```python
from build123d import *

# Parameters (mm, degrees)
SKETCH1_R           = 3.739497694
SKETCH1_R_2         = 2.032
BOSS_EXTRUDE1_DEPTH = 6.35
SKETCH2_R           = 6.5
CUT_EXTRUDE1_DEPTH  = 3.175
FILLET1_R           = 3.175
FILLET2_R           = 0.396875


with BuildPart() as part:
    # Sketch1 → Boss-Extrude1 (new, symmetric)
    with BuildSketch(Plane(origin=(0, 0, 0), x_dir=(0, 0, -1), z_dir=(1, 0, 0))):
        with BuildLine():
            Line((-5.55625, 0), (-5.55625, 28.575))
            ThreePointArc((-5.55625, 28.575), (0, 34.13125), (5.55625, 28.575))
            Line((5.55625, 28.575), (5.55625, 0))
            ThreePointArc((5.55625, 0), (0, -5.55625), (-5.55625, 0))
        make_face()
        Circle(SKETCH1_R, mode=Mode.SUBTRACT)
        with Locations((0, 28.575)):
            Circle(SKETCH1_R_2, mode=Mode.SUBTRACT)
    extrude(amount=BOSS_EXTRUDE1_DEPTH, both=True)

    # Sketch2 → Cut-Extrude1 (cut, symmetric)
    with BuildSketch(Plane(origin=(0, 0, 0), x_dir=(0, 0, -1), z_dir=(1, 0, 0))):
        with Locations((0, 28.575)):
            Circle(SKETCH2_R)
    extrude(amount=CUT_EXTRUDE1_DEPTH, both=True, mode=Mode.SUBTRACT)

    # Fillet1
    fillet1_edges = [part.edges().sort_by_distance(p)[0] for p in [
        (0, 25.20185815, 5.55625),
        (0, 25.20185815, -5.55625),
    ]]
    fillet(fillet1_edges, radius=FILLET1_R)

    # Fillet2
    fillet2_edges = [part.edges().sort_by_distance(p)[0] for p in [
        (6.35, 34.13125, 0),
        (6.35, 14.2875, 5.55625),
        (3.175, 23.886309526, -5.55625),
        (3.175, 34.13125, 0),
        (3.175, 23.886309526, 5.55625),
        (-3.175, 23.886309526, -5.55625),
        (-3.175, 34.13125, 0),
        (-3.175, 23.886309526, 5.55625),
        (6.35, -5.55625, 0),
        (-6.35, 14.2875, 5.55625),
        (-6.35, 34.13125, 0),
        (-6.35, 14.2875, -5.55625),
        (-6.35, -5.55625, 0),
        (6.35, 14.2875, -5.55625),
    ]]
    fillet(fillet2_edges, radius=FILLET2_R)


solid = part.part
```
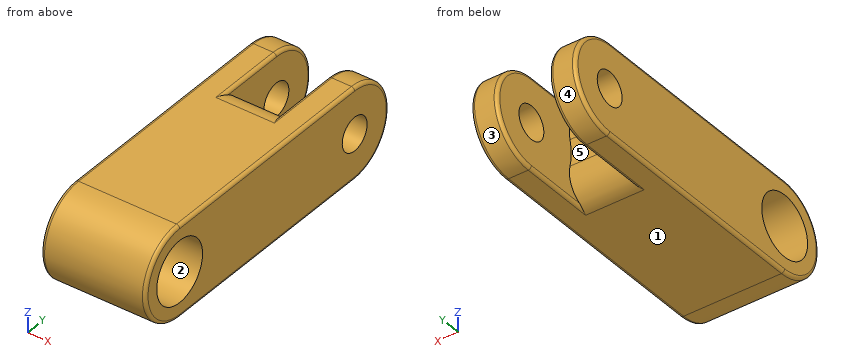
The listing builds one solid part. Answer for the finished solid, in the listing's coordinates (mm). Face numbers are marked on the shaded views. A direction names the side the tool comes from. Give positions to 0.01 mm unless a question says otherwise; leave off trailing zeros. Write each loop counter-clockwise with the first axis right and the second up, starting at its lowest first coordinate (ties: lowest second). Pieces come first, ordered by that corner, then holes. Notation, with made-up numbers: (87, 56) -> (120, 56) arc R15 cw to (120, 68) -> close; hole circle Ø6 at (79, -9.5). An arc over 180 degrees is marked (long way). Use one line per item in the form item = value.
1) Straight lines are drawn through the part: probe 1 along Y at (x, z) = (5.2, 0); probe 2 along Y at (x, z) = (0, 0) (1 decimal); probe 3 along X at (y, z) = (28, -3.5) (3 decimals). For each, find the intervals that lie inside material, in ascending order.
Result:
probe_1 = -5.56 to -3.74, 3.74 to 26.54, 30.61 to 34.13
probe_2 = -5.6 to -3.7, 3.7 to 22.1
probe_3 = -6.35 to -3.175, 3.175 to 6.35
2) A tool of negligible diameter and unlimited length cuts with its end or side. For the marked faces 4 and 5, from which of +Z, -Z, +X, -X, +Y, -Y can it reach the whole face along a straight path? Write none if from no direction.
Result:
face_4 = +X, -X, +Y
face_5 = +Y
3) Section A-A on z = 0 is taken. Count the separate pieces of the cut face and the enclosed holes in it, plus the area to 3 significant figures.
Result:
separate_pieces = 4
enclosed_holes = 0
area = 306 mm²
4) For a pull along Z with two mould halves and no side action, classify the marked faces 1, 2 and 3 as +Z half, -Z half, draft (parallel to the pull), parting line (faces both ways), or undercut.
Result:
face_1 = -Z half
face_2 = undercut
face_3 = parting line
5) Each of these flat-tipped pins is pushed along its axis until it touches: P1, Ø3.5, axis at y = 28.575, z = 0, coming from the +X side; P2, Ø4, axis at x = 0, z = 0.5, coming from the +Y side; P3, Ø2, axis at x = -2.5, z = 4, coming from the +Y side; P4, Ø2, axis at x = 4, z = -2, coming from the -Y side. Where does it stop, or does it pass through?
Result:
P1 = through
P2 = 22.37
P3 = 32.83
P4 = -5.47
6) Section C-C on x = -5.25 is taken. Write down the section's boundary in (y, z) (1 decimal), plus the area to 3 significant figures.
Result:
outline = (0, -5.6) -> (28.6, -5.6) arc R5.6 ccw to (28.6, 5.6) -> (0, 5.6) arc R5.6 ccw to start; hole circle Ø7.5 at (0, 0); hole circle Ø4.1 at (28.6, 0)
area = 358 mm²
